Here's how the part is built. I have some questions about the finished solid (model axes, mm). Face numbers are marked on the shaded views. Round coordinates to 2 decimals unless told otherwise and drop trailing zeros. Write each loop counter-clockwise with the first axis right and the second up, starting at its lowest first coordinate (ties: lowest second). Pieces come first, ordered by that corner, then holes. Notation, with made-up numbers: M -10.75,-12.5 L 5.25,-12.5 A22 cw 5.25,-2.5 Z; hole C -36,32 d5. An arc over 180 degrees is marked long. Write item = value, one per line. Start each with the question number.
(1) I want a section at A-A (y = 0). List the corners of the cut face in (x, z) for me.
(2) Will this pin go through, and if not, where does the flat tip stop? pin 1 Ø6 at (x, z) = (27.5, -8) entering from +Y.
(3) I need wall thicknesses on line 1 along Y through (x, z) = (0, -7); line 2 along X through (y, z) = (4.5, -3.25); line 3 along X through (y, z) = (-11, -6). Which ranges of each line are inside material? Lowest first, please.
(4) I want a section at B-B (z = -8.5). List the corners of the cut face in (x, y) for me.
(5) If we mould it in two halves opening along X, with no side actions, what happens to the marked faces 1, 2, 3 and 4? For each: released by +X, released by -X, zero draft, split by the parting line, or undercut.
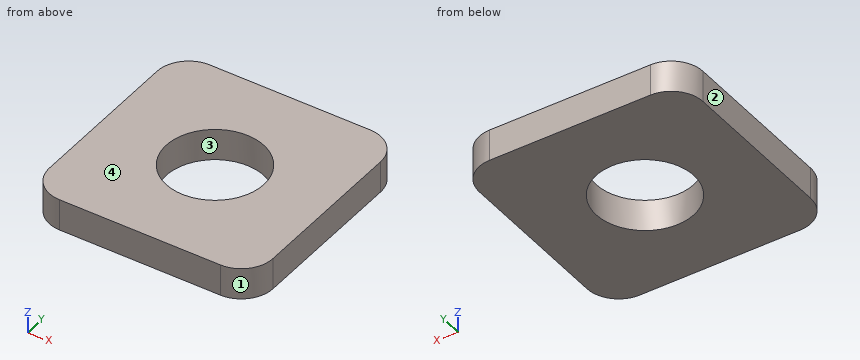
```python
from build123d import *

# Parameters (mm, degrees)
IZIM1_W            = 71
IZIM1_H            = 71
IZIM1_R            = 15.5
TABAN_FLAN_1_DEPTH = 10
RADYUS1_R          = 10


# Sheet-metal steps are written as plain solids
with BuildPart() as part:
    # Çizim1 → Taban-Flanş1 (new body)
    with BuildSketch(Plane.XY):
        Rectangle(IZIM1_W, IZIM1_H)
        Circle(IZIM1_R, mode=Mode.SUBTRACT)
    extrude(amount=-TABAN_FLAN_1_DEPTH)

    # Radyus1
    radyus1_edges = [part.edges().sort_by_distance(p)[0] for p in [
        (35.5, -35.5, -5),
        (-35.5, -35.5, -5),
        (-35.5, 35.5, -5),
        (35.5, 35.5, -5),
    ]]
    fillet(radyus1_edges, radius=RADYUS1_R)


solid = part.part
```
Returned:
q1.outline = M -35.5,-10 L -15.5,-10 L -15.5,0 L -35.5,0 Z; M 15.5,-10 L 35.5,-10 L 35.5,0 L 15.5,0 Z
q2.pin_1 = 35.5
q3.line_1 = -35.5 to -15.5, 15.5 to 35.5
q3.line_2 = -35.5 to -14.83, 14.83 to 35.5
q3.line_3 = -35.5 to -10.92, 10.92 to 35.5
q4.outline = M -35.5,-25.5 A10 ccw -25.5,-35.5 L 25.5,-35.5 A10 ccw 35.5,-25.5 L 35.5,25.5 A10 ccw 25.5,35.5 L -25.5,35.5 A10 ccw -35.5,25.5 Z; hole C 0,0 d31
q5.face_1 = released by +X
q5.face_2 = released by -X
q5.face_3 = undercut
q5.face_4 = zero draft
